Geometry check sheet. Reference: the model listing, model coordinates, mm. A direction names the side the tool comes from. Coordinates: 2 decimals unless noted, no trailing zeros. Order: outer loops, then holes, each group sorted by start corner. A loop starts at its lowest first (then second) coordinate and runs counter-clockwise, first axis right, second up. Notation, with made-up numbers: (75, -3) - (95, -3) arc R9 cw to (95, 7) - close; hole circle Ø6 at (48.5, -3.75). An arc over 180 degrees is marked (long way). Return JSON: item names as keys, results as strings. Group by question number.
Item 1: Section check B-B on x = -161. Enter the section's corners in (y, z).
Item 2: Tool access check on faces 5 (the flat face through (17, -17, 7)), 6 (the flat face through (25, -34, 8)), 7 (the cylindrical face through (-158.52, -16.76, 7.17)), 8 (the flat face through (-164, 0, 8)), 9 (the flat face through (32, 0, 8)). Record the directions out of +Z, -Z, +X, -X, +Y, -Y that give a thin tool (end or side, any length) a straight path to the whole face; none if there is none.
Item 3: Section check D-D on x = 0. Enter the section's corners in (y, z), then the cut area to 3 significant figures.
Item 4: Draft check along X on faces 1 (the flat face through (-66, 0, 8)), 2 (the cylindrical face through (31, -17, 9)), 3 (the flat face through (-66, 1, 0)), 4 (the flat face through (38.5, -17, 8)). Enter one of: pulls with the +X half, pulls with the -X half, needs draft (parallel to the pull), parting line crosses it, or undercut.
Item 5: Section check A-A on y = -20. Enter the section's corners in (x, z).
Item 6: Gauge pin test, flat ends, axial feed: pin 1 (7 mm diameter, centred on x = -20.5, z = 10, fed in from -Y); pin 2 (1.8 mm diameter, centred on x = -22, z = 10, fed in from +Y); pin 3 (8 mm diameter, centred on x = -121, z = 2.5, fed in from -Y). Record the tip position at first contact, or that the pin passes through.
Item 7: Scan lines: probe 1 along X at (y, z) = (-18.5, 7.5); probe 2 along Z at (x, y) = (-161, -9); probe 3 along X at (y, z) = (1.5, 6.75). Record each from-to range of solid material in increasing order.
Item 8: Section check C-C on z = 7.5. Give the number of separate pieces and of enclosed holes in the cut face, then the cut area to 3 significant figures.
from build123d import *

# Parameters (mm, degrees)
EXTRUDE_1_DEPTH     = 15
EXTRUDE_2_DEPTH     = 15
EXTRUDE_2_2_DEPTH   = 15
EXTRUDE_2_3_DEPTH   = 15
SKETCH_3_W          = 7
SKETCH_3_H          = 15
EXTRUDE_3_DEPTH     = 5
SKETCH_4_W          = 40
SKETCH_4_H          = 15
EXTRUDE_4_DEPTH     = 34
SKETCH_6_R          = 2.5
CUT_EXTRUDE_2_DEPTH = 34
SKETCH_7_W          = 18.5
SKETCH_7_H          = 15
CUT_EXTRUDE_3_DEPTH = 100
FILLET_1_R          = 2
FILLET_2_R          = 2


with BuildPart() as part:
    # Sketch 1 → Extrude 1 (new body)
    with BuildSketch(Plane.XY):
        with BuildLine():
            Line((-20, 0), (-17, 0))
            ThreePointArc((-17, 0), (0, 17), (17, 0))
            Line((17, 0), (20, 0))
            ThreePointArc((20, 0), (0, 20), (-20, 0))
        make_face()
    extrude(amount=EXTRUDE_1_DEPTH)



with BuildPart() as body_2:
    # Sketch 2 → Extrude 2 (new body)
    with BuildSketch(Plane.XY.offset(15)):
        with BuildLine():
            Line((-152, 0), (-149, 0))
            ThreePointArc((-149, 0), (-132, 17), (-115, 0))
            Line((-115, 0), (-112, 0))
            ThreePointArc((-112, 0), (-132, 20), (-152, 0))
        make_face()
    extrude(amount=-EXTRUDE_2_DEPTH)


with BuildPart() as body_3:
    # Sketch 2 → Extrude 2 2 (new body)
    with BuildSketch(Plane.XY.offset(15)):
        with BuildLine():
            Line((-71, 0), (-68, 0))
            ThreePointArc((-68, 0), (-88, 20), (-108, 0))
            Line((-108, 0), (-105, 0))
            ThreePointArc((-105, 0), (-88, 17), (-71, 0))
        make_face()
    extrude(amount=-EXTRUDE_2_2_DEPTH)


with BuildPart() as body_4:
    # Sketch 2 → Extrude 2 3 (new body)
    with BuildSketch(Plane.XY.offset(15)):
        with BuildLine():
            Line((-27, 0), (-24, 0))
            ThreePointArc((-24, 0), (-44, 20), (-64, 0))
            Line((-64, 0), (-61, 0))
            ThreePointArc((-61, 0), (-44, 17), (-27, 0))
        make_face()
    extrude(amount=-EXTRUDE_2_3_DEPTH)


with BuildPart() as part_1:
    add(part.part)

    add(body_2.part)  # Extrude 3 merges body 2

    add(body_3.part)  # Extrude 3 merges body 3

    add(body_4.part)  # Extrude 3 merges body 4
    # Sketch 3 → Extrude 3 (add)
    with BuildSketch(Plane.XZ):
        with Locations((-110, 7.5)):
            Rectangle(SKETCH_3_W, SKETCH_3_H)
        with Locations((-66, 7.5)):
            Rectangle(SKETCH_3_W, SKETCH_3_H)
        with Locations((-22, 7.5)):
            Rectangle(SKETCH_3_W, SKETCH_3_H)
    extrude(amount=-EXTRUDE_3_DEPTH)

    # Sketch 4 → Extrude 4 (add)
    with BuildSketch(Plane.XZ):
        with Locations((37, 7.5)):
            Rectangle(SKETCH_4_W, SKETCH_4_H)
        with Locations((-169, 7.5)):
            Rectangle(SKETCH_4_W, SKETCH_4_H)
    extrude(amount=EXTRUDE_4_DEPTH)

    # Sketch 6 → Cut-Extrude 2 (cut)
    with BuildSketch(Plane(origin=(0, 0, 0), x_dir=(1, 0, 0), z_dir=(0, 1, 0))):
        with Locations(Location((29, -7.5, 0), (0, 0, 270))):
            Circle(SKETCH_6_R)
        with Locations(Location((-161, -7.5, 0), (0, 0, 270))):
            Circle(SKETCH_6_R)
    extrude(amount=-CUT_EXTRUDE_2_DEPTH, mode=Mode.SUBTRACT)

    # Sketch 7 → Cut-Extrude 3 (cut)
    with BuildSketch(Plane(origin=(0, 0, 0), x_dir=(1, 0, 0), z_dir=(0, 1, 0))):
        with Locations((-179.75, -7.5)):
            Rectangle(SKETCH_7_W, SKETCH_7_H)
        with Locations((47.75, -7.5)):
            Rectangle(SKETCH_7_W, SKETCH_7_H)
    extrude(amount=-CUT_EXTRUDE_3_DEPTH, mode=Mode.SUBTRACT)

    # Fillet 1
    fillet_1_edges = [part_1.edges().sort_by_distance(p)[0] for p in [
        (-112.635083269, 5, 7.5),
        (-152, 0, 7.5),
        (-19.364916731, 5, 7.5),
        (-24.635083269, 5, 7.5),
        (-63.364916731, 5, 7.5),
        (-68.635083269, 5, 7.5),
        (20, 0, 7.5),
        (-107.364916731, 5, 7.5),
    ]]
    fillet(fillet_1_edges, radius=FILLET_1_R)

    # Fillet 2
    fillet_2_edges = [part_1.edges().sort_by_distance(p)[0] for p in [
        (-115, 0, 7.5),
        (-27, 0, 7.5),
        (-61, 0, 7.5),
        (-71, 0, 7.5),
        (-105, 0, 7.5),
        (-17, 0, 7.5),
    ]]
    fillet(fillet_2_edges, radius=FILLET_2_R)


solid = part_1.part
Computed:
{
 "1": {"outline": "(-34, 0) - (0, 0) - (0, 5) - (-34, 5) - close; (-34, 10) - (0, 10) - (0, 15) - (-34, 15) - close"},
 "2": {"face 5": "+Z, -Z, -Y", "face 6": "+Z, -Z, +X, -X, -Y", "face 7": "+Y, -Y", "face 8": "+Z, -Z, -X, +Y", "face 9": "+Z, -Z, +X, +Y"},
 "3": {"outline": "(17, 0) - (20, 0) - (20, 15) - (17, 15) - close", "area": "45.0 mm²"},
 "4": {"face 1": "undercut", "face 2": "undercut", "face 3": "needs draft", "face 4": "pulls with the +X half"},
 "5": {"outline": "(-170.5, 0) - (-149, 0) - (-149, 15) - (-170.5, 15) - close; (17, 0) - (38.5, 0) - (38.5, 15) - (17, 15) - close; hole circle Ø5 at (-161, 7.5); hole circle Ø5 at (29, 7.5)"},
 "6": {"pin 1": "stops at y = 0", "pin 2": "stops at y = 5", "pin 3": "stops at y = 8"},
 "7": {"probe 1": "x = -170.5 to -163.5, -158.5 to -149, 17 to 26.5, 31.5 to 38.5", "probe 2": "z = 0 to 5, 10 to 15", "probe 3": "x = -151.97 to -148.93, -115.04 to -104.96, -71.04 to -60.96, -27.04 to -16.96, 16.93 to 19.97"},
 "8": {"separate pieces": "3", "enclosed holes": "0", "area": "1,890 mm²"}
}
